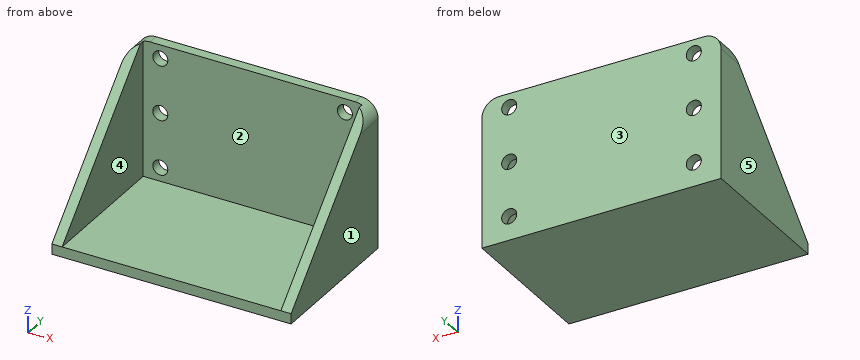
```python
from build123d import *

# Parameters (mm, degrees)
F0_W     = 64
F0_H     = 40
F0_R     = 2.2
F0_H_2   = 3
F1_DEPTH = 3
F2_DEPTH = 44
F3_SIZE  = 40
F4_R     = 5


with BuildPart() as f1:
    # F0 (on Front) → F1 (new body)
    with BuildSketch(Plane.XZ):
        Rectangle(F0_W, F0_H)
        with Locations((-27, -16)):
            Circle(F0_R, mode=Mode.SUBTRACT)
        with Locations((27, -16)):
            Circle(F0_R, mode=Mode.SUBTRACT)
        with Locations((-27, 0)):
            Circle(F0_R, mode=Mode.SUBTRACT)
        with Locations((-27, 16)):
            Circle(F0_R, mode=Mode.SUBTRACT)
        with Locations((27, 0)):
            Circle(F0_R, mode=Mode.SUBTRACT)
        with Locations((27, 16)):
            Circle(F0_R, mode=Mode.SUBTRACT)
        Polygon((32, 20), (32, -20), (32, -23), (35, -23), (35, 20), align=None)
        Polygon((-32, -23), (-32, -20), (-32, 20), (-35, 20), (-35, -23), align=None)
        with Locations((0, -21.5)):
            Rectangle(F0_W, F0_H_2)
    extrude(amount=F1_DEPTH)

    # F0 (on Front) → F2 (join)
    with BuildSketch(Plane.XZ):
        with Locations((0, -21.5)):
            Rectangle(F0_W, F0_H_2)
        Polygon((32, 20), (32, -20), (32, -23), (35, -23), (35, 20), align=None)
        Polygon((-32, -23), (-32, -20), (-32, 20), (-35, 20), (-35, -23), align=None)
    extrude(amount=F2_DEPTH)

    # F3
    f3_edges = [f1.edges().sort_by_distance(p)[0] for p in [
        (-33.5, -44, 20),
        (33.5, -44, 20),
    ]]
    chamfer(f3_edges, length=F3_SIZE)

    # F4
    f4_edges = [f1.edges().sort_by_distance(p)[0] for p in [
        (35, -2, 20),
        (-35, -2, 20),
    ]]
    fillet(f4_edges, radius=F4_R)


solid = f1.part
```
CAD build for the part. Positions are in the model's coordinates, mm. Face numbers are marked on the shaded views. A direction names the side the tool comes from. Give positions to 0.01 mm unless a question says otherwise; leave off trailing zeros. Write each loop counter-clockwise with the first axis right and the second up, starting at its lowest first coordinate (ties: lowest second). Pieces come first, ordered by that corner, then holes. Notation, with made-up numbers: M 19.5,-31.75 L 43.5,-31.75 A27 cw 43.5,-4.75 Z; hole C 48.5,57.5 d3. An arc over 180 degrees is marked long. Return JSON: item names as keys, results as strings. Group by question number.
(1) Band-saw the part on D-D (z = -11.5). Give the cut face in (x, y), and give its area (3 significant figures).
(2) Mould opens along X. For the marked faces 1, 2 and 3 say: pulls with the +X half, pulls with the -X half, needs draft (parallel to the pull), parting line crosses it, or undercut.
(3) 3-axis set-ups, long thin cutter, end or side, ignore diameter. For the marked faces 4 and 5: which of +Z, -Z, +X, -X, +Y, -Y reach the whole face in a straight line?
(4) Flat gauge pins, fed straight in: pin 1 Ø12 at (x, z) = (-1.5, -2.5) entering from -Y; pin 2 Ø4 at (x, y) = (-18, -29.5) entering from +Z. Where does each tip first touch, or does it go through?
(5) Band-saw the part on A-A (z = -16). Give the cut face in (x, y), and give its area (3 significant figures).
(6) Band-saw the part on C-C (y = -11). Give the cut face in (x, z).
(7) Drill centre lines: L1, parallel to Z at x = -27, y = -2.2; L2, parallel to X at y = -31, z = -11.5; L3, parallel to Z at x = -24, y = -38.5. Where is each one in solid material? Low to high. Write a range as [from, to].
(8) Band-saw the part on B-B (x = 27). Give the cut face in (y, z).
Entries:
{
 "1": {"outline": "M -35,-35.5 L -32,-35.5 L -32,-3 L 32,-3 L 32,-35.5 L 35,-35.5 L 35,0 L -35,0 Z", "area": "405 mm^2"},
 "2": {"face 1": "pulls with the +X half", "face 2": "undercut", "face 3": "needs draft"},
 "3": {"face 4": "+Z, -Y", "face 5": "+Z, -Z, -X, +Y, -Y"},
 "4": {"pin 1": "stops at y = -3", "pin 2": "stops at z = -20"},
 "5": {"outline": "M -35,-40 L -32,-40 L -32,-3 L -29.2,-3 L -29.2,0 L -35,0 Z; M -24.8,-3 L 24.8,-3 L 24.8,0 L -24.8,0 Z; M 29.2,-3 L 32,-3 L 32,-40 L 35,-40 L 35,0 L 29.2,0 Z", "area": "406 mm^2"},
 "6": {"outline": "M -35,-23 L 35,-23 L 35,13 L 32,13 L 32,-20 L -32,-20 L -32,13 L -35,13 Z"},
 "7": {"L1": "z = [-23, -18.2], [-13.8, -2.2], [2.2, 13.8], [18.2, 20]", "L2": "x = [-35, -32], [32, 35]", "L3": "z = [-23, -20]"},
 "8": {"outline": "M -44,-23 L 0,-23 L 0,-18.2 L -3,-18.2 L -3,-20 L -44,-20 Z; M -3,-13.8 L 0,-13.8 L 0,-2.2 L -3,-2.2 Z; M -3,2.2 L 0,2.2 L 0,13.8 L -3,13.8 Z; M -3,18.2 L 0,18.2 L 0,20 L -3,20 Z"}
}
